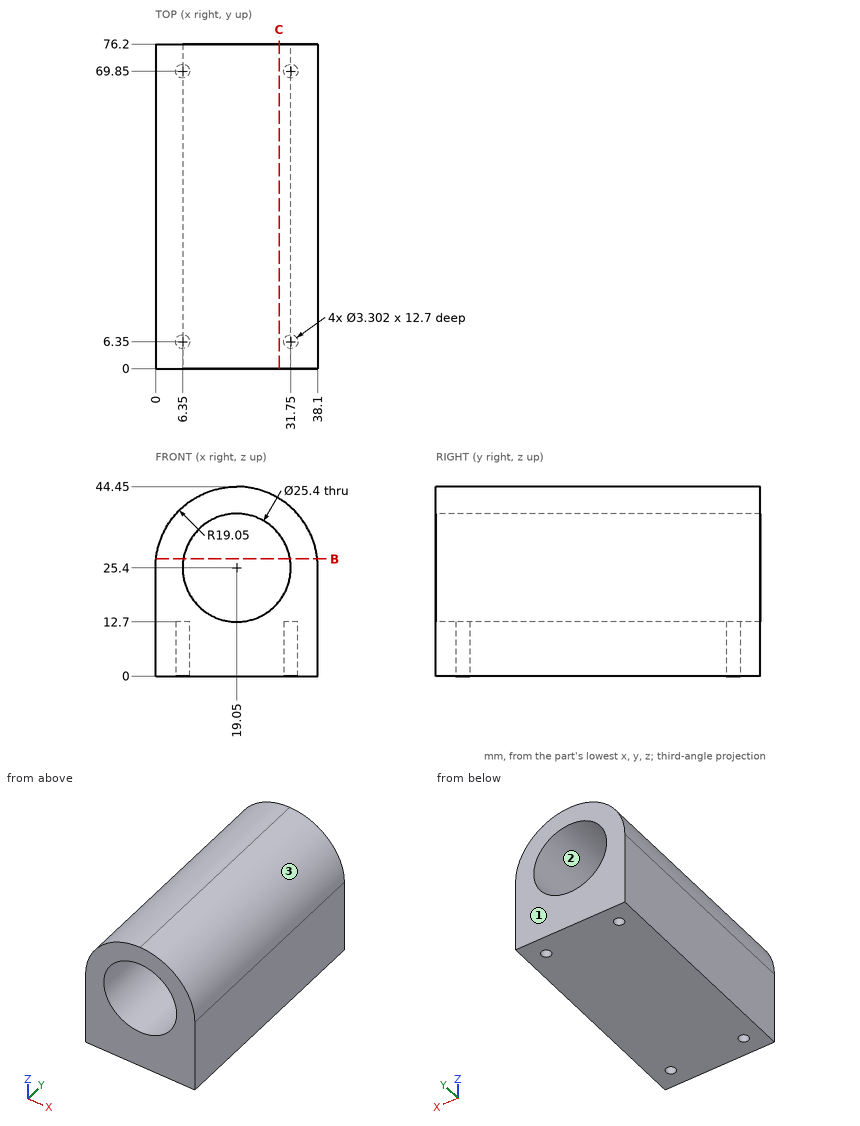
Study the drawing (mm; zero at the part's minimum x, y, z) and answer. Round coordinates to 2 decimals unless told otherwise and drop trailing zeros. Write each loop counter-clockwise with the first axis right and the second up, starting at its lowest first coordinate (ties: lowest second). Pieces come first, ordered by that corner, then holes. Notation, with made-up numbers: (4, -20) - (21, -20) arc R21 cw to (21, 5) - close; hole circle Ø7 at (42, -23). An arc over 180 degrees is marked (long way). Use a Markdown table: item, result. Add a question column.
1. The part is cut by section C-C (x = 29). Write down the section's boundary in (y, z) (3 decimals).
2. The part is cut by section B-B (z = 27.5). Write down the section's boundary in (x, y).
3. Consider line 1 (Y direction, x = 32, z = 9); line 2 (Y direction, x = 31, z = 10.5); line 3 (X direction, y = 69, z = 9). Determine where each line is inside the solid, lowest interval first.
4. For a pull along X with two mould halves and no side action, classify the marked faces 1, 2 and 3 as +X half, -X half, draft (parallel to the pull), parting line (faces both ways), or undercut.
5. Flat-ended cylindrical pins translate along their axes: P1, Ø2, axis at x = 31.75, y = 69.85, coming from the +Z side; P2, Ø2, axis at x = 9, z = 20.5, coming from the -Y side; P3, Ø10, axis at x = 24.5, y = 12, coming from the +Z side; P4, Ø2.5, axis at x = 6.35, y = 69.85, coming from the +Z side (3 decimals). Find the tip coordinate at first contact, or state that the pin passes through.
Reported:
| question | item | result |
|---|---|---|
| 1 | outline | (0, 0) - (76.2, 0) - (76.2, 17.508) - (0, 17.508) - close; (0, 33.292) - (76.2, 33.292) - (76.2, 41.645) - (0, 41.645) - close |
| 2 | outline | (0.12, 0) - (6.52, 0) - (6.52, 76.2) - (0.12, 76.2) - close; (31.58, 0) - (37.98, 0) - (37.98, 76.2) - (31.58, 76.2) - close |
| 3 | line 1 | 0 to 4.72, 7.98 to 68.22, 71.48 to 76.2 |
| 3 | line 2 | 0 to 4.88, 7.82 to 68.38, 71.32 to 76.2 |
| 3 | line 3 | 0 to 4.93, 7.77 to 30.33, 33.17 to 38.1 |
| 4 | face 1 | draft |
| 4 | face 2 | undercut |
| 4 | face 3 | +X half |
| 5 | P1 | z = 40.43 |
| 5 | P2 | through |
| 5 | P3 | z = 44.44 |
| 5 | P4 | z = 40.625 |
